from build123d import *

# Parameters (mm, degrees)
EXTRUDE_1_DEPTH = 0.5
SKETCH_2_R      = 2.5
EXTRUDE_2_DEPTH = 0.5
FILLET_1_R      = 0.25


with BuildPart() as part:
    # 草图1 → 凸台-拉伸1 (new body)
    with BuildSketch(Plane.XY):
        with BuildLine():
            Line((0, 4), (22, 4))
            ThreePointArc((22, 4), (26, 0), (22, -4))
            Line((22, -4), (0, -4))
            ThreePointArc((0, -4), (-4, 0), (0, 4))
        make_face()
    extrude(amount=EXTRUDE_1_DEPTH)

    # 草图2 → 凸台-拉伸2 (add)
    with BuildSketch(Plane.XY.offset(0.5)):
        Circle(SKETCH_2_R)
    extrude(amount=EXTRUDE_2_DEPTH)

    # 圆角1
    fillet_1_edges = [part.edges().sort_by_distance(p)[0] for p in [
        (-2.5, 0, 1),
    ]]
    fillet(fillet_1_edges, radius=FILLET_1_R)


solid = part.part
Read the model definition and answer for the solid it produces. Units are mm, in the model's axes. Coordinates: 2 decimals unless noted, no trailing zeros. Loops run counter-clockwise (first coordinate to the right, second up) from the corner with the lowest first, then second, coordinate; pieces in that order, holes last. Notation, with made-up numbers: (44.25, -28) -> (95.25, -28) arc R23 cw to (95.25, -19) -> close; hole circle Ø8 at (56, -9). An arc over 180 degrees is marked (long way). Answer in a Markdown table with one row per item.
Item 1: For a pull along X with two mould halves and no side action, classify faces 1 (the flat face through (11, 0, 0.5)), 2 (the cylindrical face through (-4, -0.1, 0.2)), 3 (the cylindrical face through (26, 0.1, 0.2)) as released by +X, released by -X, zero draft, split by the parting line, or undercut.
Returned:
| item | result |
|---|---|
| face 1 | zero draft |
| face 2 | released by -X |
| face 3 | released by +X |
Item 2: A cutting plane is placed at C-C on z = 0.25. Determine the outline of the cut face in (x, y).
Returned:
| item | result |
|---|---|
| outline | (0, -4) -> (22, -4) arc R4 ccw to (22, 4) -> (0, 4) arc R4 ccw to start |
Item 3: Straight lines are drawn through the part: line 1 along Z through (x, y) = (21, -3.5); line 2 along X through (y, z) = (1, 0.9); line 3 along X through (y, z) = (2.25, 0.7). For each, find the intervals that lie inside material, in ascending order. Write a range as [from, to].
Returned:
| item | result |
|---|---|
| line 1 | z = [0, 0.5] |
| line 2 | x = [-2.24, 2.24] |
| line 3 | x = [-1.09, 1.09] |
Item 4: A cutting plane is placed at A-A on y = 0. Determine the outline of the cut face in (x, z), plus the area to 3 significant figures.
Returned:
| item | result |
|---|---|
| outline | (-4, 0) -> (26, 0) -> (26, 0.5) -> (2.5, 0.5) -> (2.5, 0.75) arc R0.25 ccw to (2.25, 1) -> (-2.25, 1) arc R0.25 ccw to (-2.5, 0.75) -> (-2.5, 0.5) -> (-4, 0.5) -> close |
| area | 17.5 mm^2 |
Item 5: A cutting plane is placed at B-B on x = 8.25. Determine the outline of the cut face in (y, z).
Returned:
| item | result |
|---|---|
| outline | (-4, 0) -> (4, 0) -> (4, 0.5) -> (-4, 0.5) -> close |
